from build123d import *

# Parameters (mm, degrees)
F0_W      = 36.7
F0_H      = 7
F1_DEPTH  = 4
F3_R      = 0.75
F4_DEPTH  = 25
F5_R      = 1.99999
F6_R      = 0.75
F7_DEPTH  = 25
F8_R      = 1.5
F9_R      = 0.75
F10_DEPTH = 2.5
F11_DEPTH = 25


# Not quite as in the source:
# - a fillet or chamfer is up to 0.001 mm smaller than in the source, because OpenCascade refuses the exact size


with BuildPart() as f1:
    # F0 (on Top) → F1 (new body)
    with BuildSketch(Plane.XY):
        with Locations((-18.35, -3.5)):
            Rectangle(F0_W, F0_H)
    extrude(amount=F1_DEPTH)

    # F3 (on face) → F4 (cut)
    with BuildSketch(Plane(origin=(0, 0, 0), x_dir=(-1, 0, 0), z_dir=(0, 1, 0))):
        with Locations((2, 2)):
            Circle(F3_R)
    extrude(amount=-F4_DEPTH, mode=Mode.SUBTRACT)

    # F5 (radius 2 in the source; OpenCascade refuses exactly that, so slightly less here)
    f5_edges = [f1.edges().sort_by_distance(p)[0] for p in [
        (-36.7, -3.5, 0),
        (-36.7, -3.5, 4),
    ]]
    fillet(f5_edges, radius=F5_R)

    # F6 (on face) → F7 (cut)
    with BuildSketch(Plane(origin=(0, 0, 0), x_dir=(-1, 0, 0), z_dir=(0, 1, 0))):
        with Locations((34.7, 2)):
            Circle(F6_R)
    extrude(amount=-F7_DEPTH, mode=Mode.SUBTRACT)

    # F8
    f8_edges = [f1.edges().sort_by_distance(p)[0] for p in [
        (0, -3.5, 4),
        (0, -3.5, 0),
    ]]
    fillet(f8_edges, radius=F8_R)

    # F9 (on face) → F10 (cut)
    with BuildSketch(Plane.XZ.offset(7)):
        Polygon((-33.45, 1.482233047), (-33.45, 2.517766953), (-34.182233047, 3.25), (-35.217766953, 3.25), (-35.95, 2.517766953), (-35.95, 1.482233047), (-35.217766953, 0.75), (-34.182233047, 0.75), align=None)
        with Locations((-34.7, 2)):
            Circle(F9_R, mode=Mode.SUBTRACT)
    extrude(amount=-F10_DEPTH, mode=Mode.SUBTRACT)

    # F2 (on face) → F11 (cut)
    with BuildSketch(Plane.XY.offset(4)):
        Polygon((-36.7, 0), (-36.7, -1.75), (-10, 0), align=None)
        Polygon((-10, -7), (-36.7, -5.25), (-36.7, -7), align=None)
    extrude(amount=-F11_DEPTH, mode=Mode.SUBTRACT)


solid = f1.part
Here's how the part is built. I have some questions about the finished solid (model axes, mm). A direction names the side the tool comes from. Round coordinates to 2 decimals unless told otherwise and drop trailing zeros. Loops run counter-clockwise (first coordinate to the right, second up) from the corner with the lowest first, then second, coordinate; pieces in that order, holes last.
1. If we section it at C-C on x = -12.5: Write out the boundary of the cut face in (y, z), plus the area to 3 significant figures.
Answer list:
outline: (-6.84, 0) - (-0.16, 0) - (-0.16, 4) - (-6.84, 4) - close
area: 26.7 mm2
2. For P1, Ø1, axis at x = -17, z = 0.5, coming from the +Y side, with a flat end and sliding along its axis, tell me the tip position at first contact or that it passes through.
Answer list:
P1: stops at y = -0.43
3. If I drill on line 1 along X through (y, z) = (-3, 2.05); line 2 along Z through (x, y) = (-2, -1.25); line 3 along X through (y, z) = (-4.25, 1.45), over which ranges is the centre line in solid material (lowest first)?
Answer list:
line 1: x = -36.7 to -35.45, -33.95 to -2.75, -1.25 to 0
line 2: z = 0 to 1.25, 2.75 to 4
line 3: x = -36.62 to -35.21, -34.19 to -2.51, -1.49 to 0
4. We'd pull the mould along Z, two halves only. Please class faces 1 (the face through (-23.537, -0.887, 2.028)), 2 (the face through (-15, -3, 4)), 3 (the face through (-33.95, -3.01, 2.03)): +Z half, -Z half, draft (parallel to the pull), parting line (faces both ways), or undercut.
Answer list:
face 1: draft
face 2: +Z half
face 3: undercut
5. If we section it at B-B on y = -6.25: Write out the boundary of the cut face in (x, z), plus the area to 3 significant figures.
Answer list:
outline: (-21.44, 0) - (-1.5, 0) arc R1.5 ccw to (0, 1.5) - (0, 2.5) arc R1.5 ccw to (-1.5, 4) - (-21.44, 4) - close; hole circle Ø1.5 at (-2, 2)
area: 83.0 mm2
6. If we section it at A-A on x = -2: Write out the boundary of the cut face in (y, z).
Answer list:
outline: (-7, 0) - (0, 0) - (0, 1.25) - (-7, 1.25) - close; (-7, 2.75) - (0, 2.75) - (0, 4) - (-7, 4) - close
7. Which directions (+Z, -Z, +X, -X, +Y, -Y) give clear straight access to the entire face, cutting with the end or side of a thin tool? Please do faces 4 (the face through (-35, -4.5, 3)), 5 (the face through (-0.45, -3.45, 3.57)).
Answer list:
face 4: -Y
face 5: +Z, +X, +Y, -Y
8. If we section it at D-D on x = -30.5: Write out the boundary of the cut face in (y, z), plus the area to 3 significant figures.
Answer list:
outline: (-5.66, 0) - (-1.34, 0) - (-1.34, 4) - (-5.66, 4) - close
area: 17.3 mm2
